```python
from build123d import *

# Parameters (mm, degrees)
SKETCH1_R           = 125
SKETCH1_R_2         = 14.75
BOSS_EXTRUDE1_DEPTH = 6
CUT_EXTRUDE1_DEPTH  = 6
CIRPATTERN1_COUNT   = 4
SKETCH3_R           = 2.75
CUT_EXTRUDE2_DEPTH  = 10


with BuildPart() as part:
    # Sketch1 → Boss-Extrude1 (new body)
    with BuildSketch(Plane(origin=(0, 0, 0), x_dir=(1, 0, 0), z_dir=(0, 1, 0))):
        Circle(SKETCH1_R)
        Circle(SKETCH1_R_2, mode=Mode.SUBTRACT)
    extrude(amount=BOSS_EXTRUDE1_DEPTH)

    # Sketch2 → Cut-Extrude1 (cut)
    with BuildSketch(Plane(origin=(0, 6, 0), x_dir=(1, 0, 0), z_dir=(0, 1, 0))):
        with BuildLine():
            Line((-46.306580885, -72.797871526), (-67.089494394, -105.470373764))
            Line((-67.089494394, -105.470373764), (-67.089494394, -164.92916021))
            Line((-67.089494394, -164.92916021), (95.10689036, -142.696592277))
            Line((95.10689036, -142.696592277), (95.10689036, -81.115223023))
            Line((95.10689036, -81.115223023), (65.644777188, -55.987433946))
            ThreePointArc((65.644777188, -55.987433946), (5.838619266, -38.883066128), (-46.306580885, -72.797871526))
        make_face()
    cut_extrude1 = extrude(amount=-CUT_EXTRUDE1_DEPTH, mode=Mode.SUBTRACT)

    # CirPattern1: Cut-Extrude1 ×4 about axis
    cirpattern1_axis = Axis((0, 0, 0), (0, 1, 0))
    for i in range(1, CIRPATTERN1_COUNT):
        add(cut_extrude1.rotate(cirpattern1_axis, i * 360 / CIRPATTERN1_COUNT), mode=Mode.SUBTRACT)

    # Sketch3 → Cut-Extrude2 (cut)
    with BuildSketch(Plane(origin=(0, 6, 0), x_dir=(1, 0, 0), z_dir=(0, 1, 0))):
        with Locations((-1.313428811, -23.463267137)):
            Circle(SKETCH3_R)
        with Locations((19.663070991, -12.869096285)):
            Circle(SKETCH3_R)
        with Locations((20.976499803, 10.594170852)):
            Circle(SKETCH3_R)
        with Locations((1.313428812, 23.463267137)):
            Circle(SKETCH3_R)
        with Locations((-19.663070991, 12.869096286)):
            Circle(SKETCH3_R)
        with Locations((-20.976499802, -10.594170852)):
            Circle(SKETCH3_R)
    extrude(amount=-CUT_EXTRUDE2_DEPTH, mode=Mode.SUBTRACT)


solid = part.part
```
For this review, take the finished solid that the model builds, in its own axes (mm). A direction names the side the tool comes from. Give positions to 0.01 mm unless a question says otherwise; leave off trailing zeros. Write each loop counter-clockwise with the first axis right and the second up, starting at its lowest first coordinate (ties: lowest second). Pieces come first, ordered by that corner, then holes.
Item 1: Insertion check: P1, Ø3, axis at x = 2, y = 2, coming from the +Z side; P2, Ø1.5, axis at x = 33, y = 1.5, coming from the -Z side; P3, Ø1, axis at y = 1, z = 73, coming from the -X side. Each pin has a flat end and moves straight along its axis. Give the tip position at first contact, or say it passes through.
Item 2: Take a section at B-B (z = 0). Give the boundary of the cut face in (x, y).
Item 3: Take a section at A-A (x = 51.5). Give the boundary of the cut face in (y, z), and give its area (3 significant figures).
Item 4: The part is to be moulded in two halves that separate along Z. For faces 4 (the face through (-74.38, 2.96, 100.46)), 5 (the face through (-38.755, 3.042, 6.727)), 6 (the face through (-100.46, 2.96, -74.38)), say which applies: +Z half, -Z half, draft (parallel to the pull), parting line (faces both ways), or undercut.
Item 5: Wall thickness on probe 1 along X at (y, z) = (5.65, -12); probe 2 along Z at (x, y) = (0, 2.2); probe 3 along Z at (x, y) = (79, 2.25): over which ranges is each line inside the solid? List them lowest first.
Item 6: Take a section at C-C (y = 1.4). Give the boundary of the cut face in (x, z).
Item 7: Machinability: for faces 1 (the face through (80.582, 3.042, 68.727)), 2 (the face through (56.553, 3.042, -88.905)), 3 (the face through (68.727, 3.042, -80.582)), which of the approach directions +Z, -Z, +X, -X, +Y, -Y give a long, thin tool a straight path to every point of the face, cutting with its end or side? Answer none if there is none.
Established:
1. P1: stops at z = 39.88
1. P2: stops at z = -57.81
1. P3: stops at x = -62.69
2. outline: (-40, 0) - (-14.75, 0) - (-14.75, 6) - (-40, 6) - close; (14.75, 0) - (40, 0) - (40, 6) - (14.75, 6) - close
3. outline: (0, -80.96) - (6, -80.96) - (6, -59.83) - (0, -59.83) - close; (0, 25.88) - (6, 25.88) - (6, 46.47) - (0, 46.47) - close
3. area: 250 mm2
4. face 4: +Z half
4. face 5: undercut
4. face 6: -Z half
5. probe 1: x = -43.87 to -22.27, -17.05 to -8.58, 8.58 to 18.61, 23.34 to 38.22
5. probe 2: z = -40 to -25.88, -21.05 to -14.75, 14.75 to 21.05, 25.88 to 40
5. probe 3: z = -96.87 to -92.63, 50.25 to 67.38
6. outline: (-105.47, -67.09) arc R125 ccw to (-95.11, -81.12) - (-65.64, -55.99) arc R75 cw to (46.31, -72.8) - (67.09, -105.47) arc R125 ccw to (81.12, -95.11) - (55.99, -65.64) arc R75 cw to (72.8, 46.31) - (105.47, 67.09) arc R125 ccw to (95.11, 81.12) - (65.64, 55.99) arc R75 cw to (-46.31, 72.8) - (-67.09, 105.47) arc R125 ccw to (-81.12, 95.11) - (-55.99, 65.64) arc R75 cw to (-72.8, -46.31) - close; hole circle Ø5.5 at (-20.98, 10.59); hole circle Ø5.5 at (-19.66, -12.87); hole circle Ø29.5 at (0, 0); hole circle Ø5.5 at (-1.31, 23.46); hole circle Ø5.5 at (1.31, -23.46); hole circle Ø5.5 at (19.66, 12.87); hole circle Ø5.5 at (20.98, -10.59)
7. face 1: +Z, +Y, -Y
7. face 2: -Z, +Y, -Y
7. face 3: +X, +Y, -Y
